Geometry: see drawing. Coordinates: mm, zero at the bounding-box minimum. A direction names the side the tool comes from. Coordinates: 2 decimals unless noted, no trailing zeros. Loops run counter-clockwise (first coordinate to the right, second up) from the corner with the lowest first, then second, coordinate; pieces in that order, holes last. Notation, with made-up numbers: (11, -0.5) - (19, -0.5) arc R18 cw to (19, 23.5) - close; hole circle Ø11 at (-23, 1.25). An arc over 180 degrees is marked (long way). Use one line per item in the form item = value.
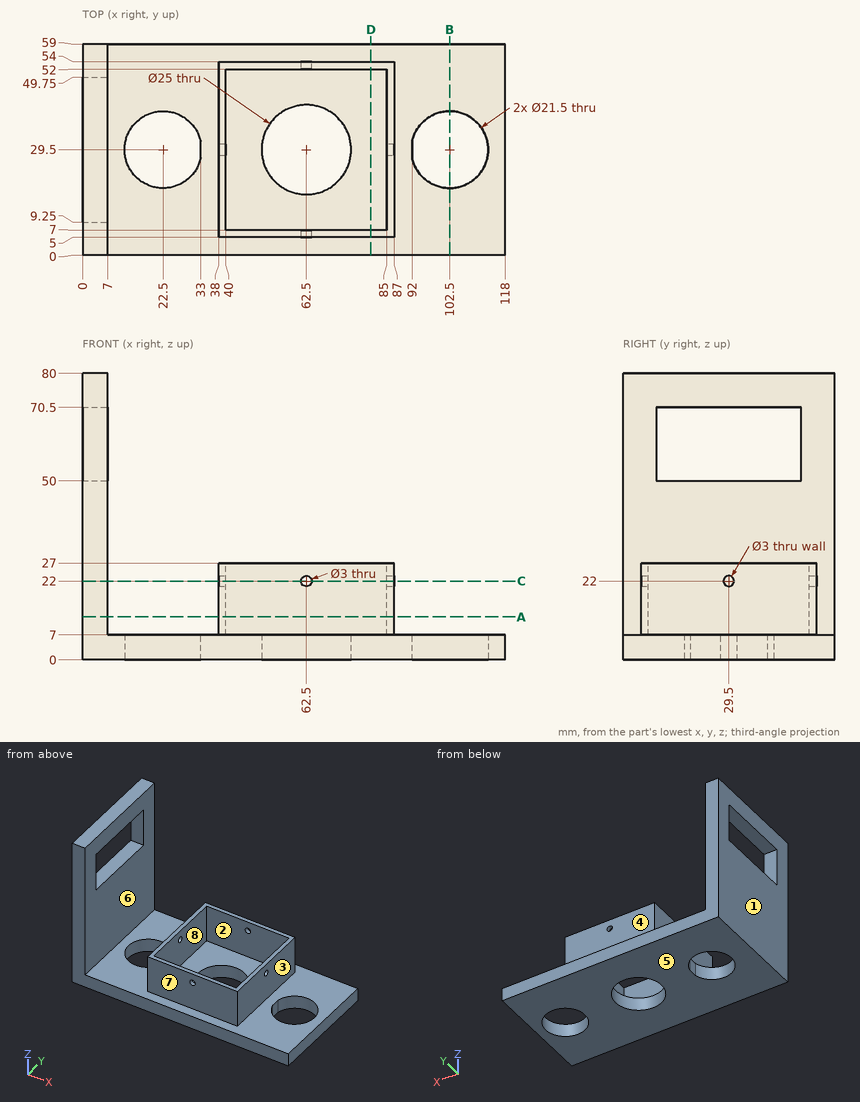
Q1. Cut plane B-B, the plane x = 102.5. Return loops of the section in (y, z).
Check values:
outline = (0, 0) - (18.75, 0) - (18.75, 7) - (0, 7) - close; (40.25, 0) - (59, 0) - (59, 7) - (40.25, 7) - close
Q2. Ray query, line 1 along X through (y, z) = (51.5, 8.5); line 2 along X through (y, z) = (29, 3); line 3 along Z through (x, y) = (62.5, 52.8). Return the intervals inside material, ascending. Write a range as [from, to].
Check values:
line_1 = [0, 7], [38, 40], [85, 87]
line_2 = [0, 11.76], [33, 50.01], [74.99, 92], [113.24, 118]
line_3 = [0, 20.5], [23.5, 27]
Q3. Pull-direction query (Y, two-part tool) for the marked faces 6, 7 and 8; classes: pulls with the +Y half, pulls with the -Y half, needs draft (parallel to the pull), parting line crosses it, or undercut.
Check values:
face_6 = needs draft
face_7 = pulls with the -Y half
face_8 = undercut
Q4. Cut plane C-C, the plane z = 22. Return loops of the section in (x, y).
Check values:
outline = (0, 0) - (7, 0) - (7, 59) - (0, 59) - close; (38, 5) - (61, 5) - (61, 7) - (40, 7) - (40, 28) - (38, 28) - close; (38, 31) - (40, 31) - (40, 52) - (61, 52) - (61, 54) - (38, 54) - close; (64, 5) - (87, 5) - (87, 28) - (85, 28) - (85, 7) - (64, 7) - close; (64, 52) - (85, 52) - (85, 31) - (87, 31) - (87, 54) - (64, 54) - close
Q5. Set-up query: the marked faces 1, 2, 3, 4 and 5. Return all of +Z, -Z, +X, -X, +Y, -Y with unobstructed straight access to the full face (end or side cutting, diameter ignored); none if empty.
Check values:
face_1 = +Z, -Z, -X, +Y, -Y
face_2 = +Z
face_3 = +Z, +X, +Y, -Y
face_4 = +Z, +X, +Y
face_5 = -Z, +X, -X, +Y, -Y
Q6. Cut plane A-A, the plane z = 12. Return loops of the section in (x, y).
Check values:
outline = (0, 0) - (7, 0) - (7, 59) - (0, 59) - close; (38, 5) - (87, 5) - (87, 54) - (38, 54) - close; hole (40, 7) - (85, 7) - (85, 52) - (40, 52) - close
Q7. Cut plane D-D, the plane x = 80.5. Return loops of the section in (y, z), then the cut area to 3 significant figures.
Check values:
outline = (0, 0) - (59, 0) - (59, 7) - (54, 7) - (54, 27) - (52, 27) - (52, 7) - (7, 7) - (7, 27) - (5, 27) - (5, 7) - (0, 7) - close
area = 493 mm²
Q8. First-contact query: P1, Ø24.5, axis at x = 63, y = 24.5, coming from the +Z side; P2, Ø4, axis at x = 62.5, z = 22, coming from the -Y side; P3, Ø12, axis at x = 45, y = 25.5, coming from the +Z side; P4, Ø10, axis at x = 39, z = 36.5, coming from the +Y side. Flat tips, straight axial feed; report the tip coordinate or a pass-through.
Check values:
P1 = 7
P2 = 5
P3 = 27
P4 = through
